Could you check a few things on this model? Use its own coordinates, in mm. Face numbers are marked on the shaded views. Give positions to 0.01 mm unless a question says otherwise; leave off trailing zeros. Write each loop counter-clockwise with the first axis right and the second up, starting at its lowest first coordinate (ties: lowest second). Pieces come first, ordered by that corner, then holes. Notation, with made-up numbers: M -1,-16 L 16,-16 A19 cw 16,-12 Z; hole C 63,13 d1. An arc over 180 degrees is marked long. Answer as a JSON object with one key per item and string values. Group by question number.
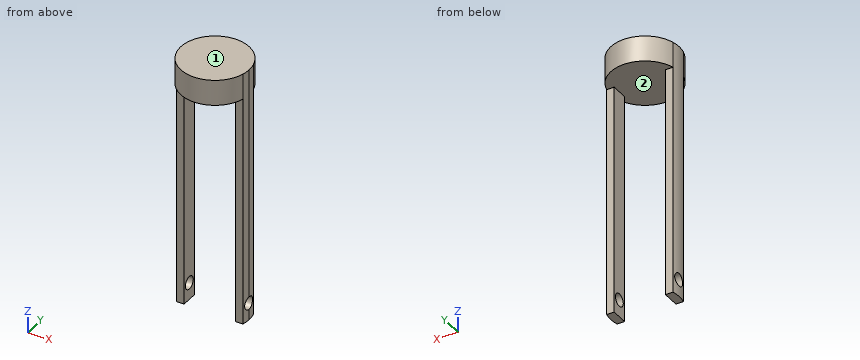
```python
from build123d import *

# Parameters (mm, degrees)
BOSS_EXTRUDE1_DEPTH     = 38.1
BOSS_EXTRUDE2_DEPTH     = 381
CUT_EXTRUDE1_DEPTH      = 395.518504002
CUT_EXTRUDE1_DEPTH_BACK = 395.518504002
SKETCH2_R               = 9.525


with BuildPart() as part:
    # Sketch1 → Boss-Extrude1 (new body)
    with BuildSketch(Plane.XY):
        with BuildLine():
            Line((38.1, 12.7), (49.186888497, 12.7))
            ThreePointArc((49.186888497, 12.7), (0, 50.8), (-49.186888497, 12.7))
            Line((-49.186888497, 12.7), (-38.1, 12.7))
            Line((-38.1, 12.7), (-38.1, -12.7))
            Line((-38.1, -12.7), (-49.186888497, -12.7))
            ThreePointArc((-49.186888497, -12.7), (0, -50.8), (49.186888497, -12.7))
            Line((49.186888497, -12.7), (38.1, -12.7))
            Line((38.1, -12.7), (38.1, 12.7))
        make_face()
    extrude(amount=-BOSS_EXTRUDE1_DEPTH)

    # Sketch1_3 → Boss-Extrude2 (add)
    with BuildSketch(Plane.XY):
        with BuildLine():
            Line((-38.1, 12.7), (-49.186888497, 12.7))
            ThreePointArc((-49.186888497, 12.7), (-50.8, 0), (-49.186888497, -12.7))
            Line((-49.186888497, -12.7), (-38.1, -12.7))
            Line((-38.1, -12.7), (-38.1, 12.7))
        make_face()
        with BuildLine():
            ThreePointArc((50.8, 0), (50.39510857, 6.401018058), (49.186888497, 12.7))
            Line((49.186888497, 12.7), (38.1, 12.7))
            Line((38.1, 12.7), (38.1, -12.7))
            Line((38.1, -12.7), (49.186888497, -12.7))
            ThreePointArc((49.186888497, -12.7), (50.39510857, -6.401018058), (50.8, 0))
        make_face()
    extrude(amount=-BOSS_EXTRUDE2_DEPTH)

    # Sketch2 → Cut-Extrude1 (cut, two sides: drawn at the far end of the back side and taken through both)
    with BuildSketch(Plane(origin=(-38.1, 0, 0), x_dir=(0, 0, -1), z_dir=(1, 0, 0)).offset(-CUT_EXTRUDE1_DEPTH_BACK)):
        with Locations((355.6, 0)):
            Circle(SKETCH2_R)
    extrude(amount=CUT_EXTRUDE1_DEPTH + CUT_EXTRUDE1_DEPTH_BACK, mode=Mode.SUBTRACT)


solid = part.part
```
1) If we section it at B-B, the plane z = -355.6: List the corners of the cut face in (x, y) for me (3 decimals), plus the area to 3 significant figures.
2) We'd pull the mould along X, two halves only. Please class the marked faces 1 and 2: released by +X, released by -X, zero draft, split by the parting line, or undercut.
3) If we section it at D-D, the plane y = -44: List the corners of the cut face in (x, z) for me.
4) If we section it at C-C, the plane x = -22.5: List the corners of the cut face in (y, z) for me.
5) If we section it at A-A, the plane z = -234: List the corners of the cut face in (x, y) for me.
6) Please list where these lines run through material, in increasing order: line 1 along Z through (x, y) = (46.5, 0) (3 decimals); line 2 along Y through (x, z) = (46, -355.6) (3 decimals); line 3 along Z through (x, y) = (-11, 36). Write a range as from..to.
7) I'm going to push flat-ended pins straight in: pin 1 (5 mm diameter, centred on x = 3.5, y = -29.5, fed in from +Z); pin 2 (12 mm diameter, centred on x = 42, z = -264.5, fed in from -Y); pin 3 (20.5 mm diameter, centred on y = 3.5, z = -165, fed in from -X); pin 4 (4 mm diameter, centred on x = -20, y = 28.5, fed in from -Z). Where does each tip first touch, or does it pass through?
Taken from the geometry:
{
 "1": {"outline": "M -49.899,-9.525 A50.8 ccw -49.187,-12.7 L -38.1,-12.7 L -38.1,-9.525 Z; M -49.899,9.525 L -38.1,9.525 L -38.1,12.7 L -49.187,12.7 A50.8 ccw Z; M 38.1,-12.7 L 49.187,-12.7 A50.8 ccw 49.899,-9.525 L 38.1,-9.525 Z; M 38.1,9.525 L 49.899,9.525 A50.8 ccw 49.187,12.7 L 38.1,12.7 Z", "area": "146 mm²"},
 "2": {"face 1": "zero draft", "face 2": "undercut"},
 "3": {"outline": "M -25.39,-38.1 L 25.39,-38.1 L 25.39,0 L -25.39,0 Z"},
 "4": {"outline": "M -45.55,-38.1 L 45.55,-38.1 L 45.55,0 L -45.55,0 Z"},
 "5": {"outline": "M -49.19,-12.7 L -38.1,-12.7 L -38.1,12.7 L -49.19,12.7 A50.8 ccw Z; M 38.1,-12.7 L 49.19,-12.7 A50.8 ccw 49.19,12.7 L 38.1,12.7 Z"},
 "6": {"line 1": "-381..-365.125, -346.075..0", "line 2": "-12.7..-9.525, 9.525..12.7", "line 3": "-38.1..0"},
 "7": {"pin 1": "z = 0", "pin 2": "y = -12.7", "pin 3": "x = -50.8", "pin 4": "z = -38.1"}
}
